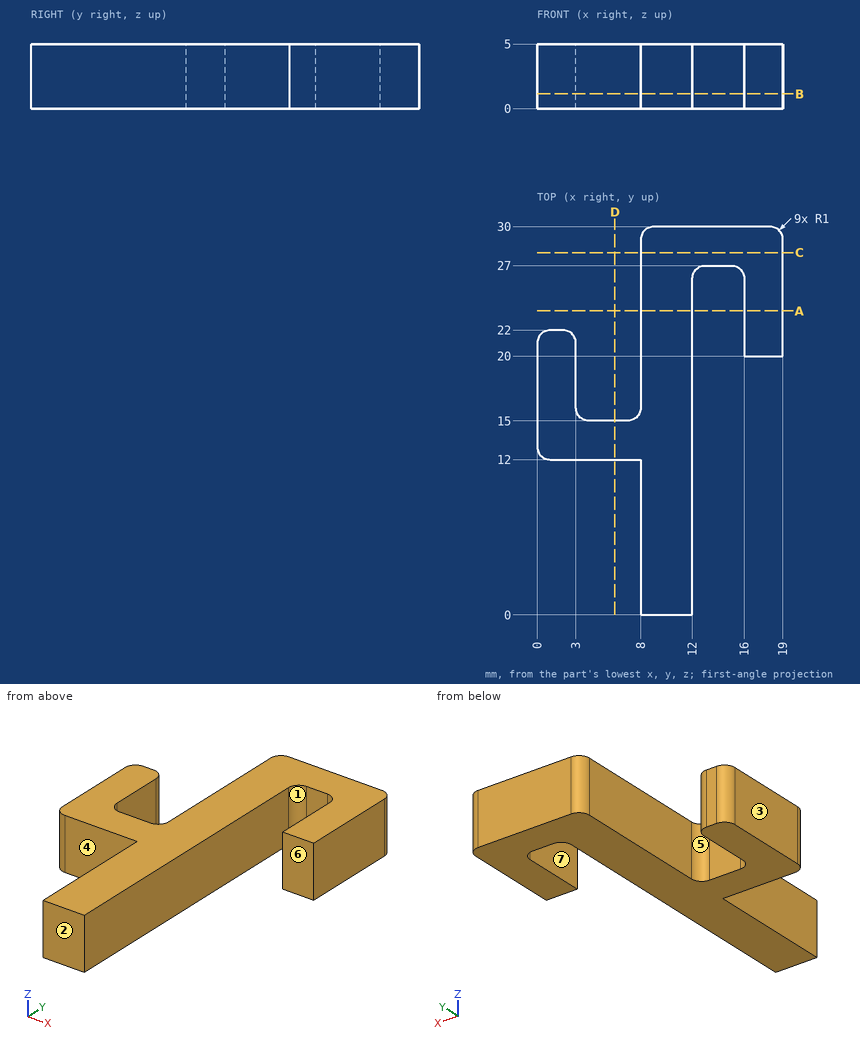
Answer from the drawing. Dimensions are ordinates in mm from the lowest x, y and z of the part. A direction names the side the tool comes from. Coordinates: 2 decimals unless noted, no trailing zeros. Loops run counter-clockwise (first coordinate to the right, second up) from the corner with the lowest first, then second, coordinate; pieces in that order, holes last. Notation, with made-up numbers: (87.25, -22) -> (108.25, -22) arc R33 cw to (108.25, 14) -> close; hole circle Ø3 at (-16, 46). An arc over 180 degrees is marked (long way). Answer in a Markdown table with one row per item.
Item 1: For a pull along X with two mould halves and no side action, classify the marked faces 1, 2 and 3 as released by +X, released by -X, zero draft, split by the parting line, or undercut.
Returned:
| item | result |
|---|---|
| face 1 | undercut |
| face 2 | zero draft |
| face 3 | released by -X |
Item 2: For the marked faces 4, 5, 6 and 7, determine the directions among +Z, -Z, +X, -X, +Y, -Y from which every point of the face is accessible in a straight line to the end or side of a thin tool.
Returned:
| item | result |
|---|---|
| face 4 | +Z, -Z, -X, -Y |
| face 5 | +Z, -Z, +Y |
| face 6 | +Z, -Z, +X, -Y |
| face 7 | +Z, -Z, -Y |
Item 3: Straight lines are drawn through the part: line 1 along X through (y, z) = (19, 2.55); line 2 along X through (y, z) = (23, 4.35); line 3 along X through (y, z) = (4, 0.3). For each, find the intervals that lie inside material, in ascending order. Write a range as [from, to].
Returned:
| item | result |
|---|---|
| line 1 | x = [0, 3], [8, 12] |
| line 2 | x = [8, 12], [16, 19] |
| line 3 | x = [8, 12] |
Item 4: Each of these flat-tipped pins is pushed along its axis until it touches: P1, Ø0.9, axis at x = 17, z = 3.5, coming from the -Y side; P2, Ø8, axis at x = 13, y = 19.5, coming from the +Z side; P3, Ø1.5, axis at x = 6.5, y = 24.5, coming from the +Z side; P4, Ø2.5, axis at x = 4.5, z = 2.5, coming from the -Y side. Where does it stop, or does it pass through?
Returned:
| item | result |
|---|---|
| P1 | stops at y = 20 |
| P2 | stops at z = 5 |
| P3 | passes through |
| P4 | stops at y = 12 |
Item 5: A cutting plane is placed at B-B on z = 1.15. Determine the outline of the cut face in (x, y).
Returned:
| item | result |
|---|---|
| outline | (0, 13) arc R1 ccw to (1, 12) -> (8, 12) -> (8, 0) -> (12, 0) -> (12, 26) arc R1 cw to (13, 27) -> (15, 27) arc R1 cw to (16, 26) -> (16, 20) -> (19, 20) -> (19, 29) arc R1 ccw to (18, 30) -> (9, 30) arc R1 ccw to (8, 29) -> (8, 16) arc R1 cw to (7, 15) -> (4, 15) arc R1 cw to (3, 16) -> (3, 21) arc R1 ccw to (2, 22) -> (1, 22) arc R1 ccw to (0, 21) -> close |
Item 6: A cutting plane is placed at A-A on y = 23.5. Determine the outline of the cut face in (x, z), plus the area to 3 significant figures.
Returned:
| item | result |
|---|---|
| outline | (8, 0) -> (12, 0) -> (12, 5) -> (8, 5) -> close; (16, 0) -> (19, 0) -> (19, 5) -> (16, 5) -> close |
| area | 35.0 mm^2 |
Item 7: A cutting plane is placed at D-D on x = 6. Determine the outline of the cut face in (y, z), plus the area to 3 significant figures.
Returned:
| item | result |
|---|---|
| outline | (12, 0) -> (15, 0) -> (15, 5) -> (12, 5) -> close |
| area | 15.0 mm^2 |
Item 8: A cutting plane is placed at C-C on y = 28. Determine the outline of the cut face in (x, z), plus the area to 3 significant figures.
Returned:
| item | result |
|---|---|
| outline | (8, 0) -> (19, 0) -> (19, 5) -> (8, 5) -> close |
| area | 55.0 mm^2 |
